Build history of the part. All positions in model axes, mm. Face numbers are marked on the shaded views. Give positions to 0.01 mm unless a question says otherwise; leave off trailing zeros. Write each loop counter-clockwise with the first axis right and the second up, starting at its lowest first coordinate (ties: lowest second). Pieces come first, ordered by that corner, then holes. Notation, with made-up numbers: M 9.25,58.25 L 28.25,58.25 A22 cw 28.25,64.25 Z; hole C 13.5,-10 d8. An arc over 180 degrees is marked long. One line per item, written item: value. Start each with the question number.
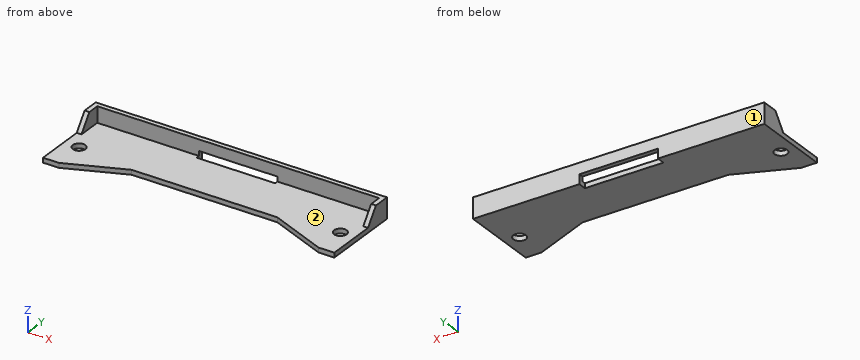
from build123d import *

# Parameters (mm, degrees)
SKETCH1_W           = 184
SKETCH1_H           = 50
SKETCH1_R           = 4
BOSS_EXTRUDE2_DEPTH = 3
SKETCH2_W           = 184
SKETCH2_H           = 3
BOSS_EXTRUDE3_DEPTH = 20
BOSS_EXTRUDE4_DEPTH = 3
BOSS_EXTRUDE5_DEPTH = 3
SKETCH5_W           = 49.622419658
SKETCH5_H           = 10.386730574
CUT_EXTRUDE3_DEPTH  = 6
SKETCH7_W           = 184
SKETCH7_H           = 10
CUT_EXTRUDE5_DEPTH  = 16
CUT_EXTRUDE7_DEPTH  = 16


with BuildPart() as part:
    # Sketch1 → Boss-Extrude2 (new body)
    with BuildSketch(Plane.XY):
        with Locations((92, 25)):
            Rectangle(SKETCH1_W, SKETCH1_H)
        with Locations((9.5, 20)):
            Circle(SKETCH1_R, mode=Mode.SUBTRACT)
        with Locations((174.5, 20)):
            Circle(SKETCH1_R, mode=Mode.SUBTRACT)
    extrude(amount=BOSS_EXTRUDE2_DEPTH)

    # Sketch2 → Boss-Extrude3 (add)
    with BuildSketch(Plane.XY.offset(3)):
        with Locations((92, 48.5)):
            Rectangle(SKETCH2_W, SKETCH2_H)
    extrude(amount=BOSS_EXTRUDE3_DEPTH)

    # Sketch3 → Boss-Extrude4 (add)
    with BuildSketch(Plane.ZY):
        Polygon((23, 47), (3, 47), (3, 32), align=None)
    extrude(amount=-BOSS_EXTRUDE4_DEPTH)

    # Sketch4 → Boss-Extrude5 (add)
    with BuildSketch(Plane(origin=(184, 0, 0), x_dir=(0, 0, -1), z_dir=(1, 0, 0))):
        Polygon((-23, 47), (-3, 32), (-3, 47), align=None)
    extrude(amount=-BOSS_EXTRUDE5_DEPTH)

    # Sketch5 → Cut-Extrude3 (cut)
    with BuildSketch(Plane(origin=(0, 0, 0), x_dir=(-1, 0, 0), z_dir=(0, 0, -1))):
        with Locations((-92, 50)):
            Rectangle(SKETCH5_W, SKETCH5_H)
    extrude(amount=-CUT_EXTRUDE3_DEPTH, mode=Mode.SUBTRACT)

    # Sketch7 → Cut-Extrude5 (cut)
    with BuildSketch(Plane(origin=(0, 50, 0), x_dir=(1, 0, 0), z_dir=(0, 1, 0))):
        with Locations((92, -18)):
            Rectangle(SKETCH7_W, SKETCH7_H)
    extrude(amount=-CUT_EXTRUDE5_DEPTH, mode=Mode.SUBTRACT)

    # Sketch8 → Cut-Extrude7 (cut)
    with BuildSketch(Plane.XY.offset(3)):
        Polygon((46, 15), (10, 0), (174, 0), (138, 15), align=None)
    extrude(amount=-CUT_EXTRUDE7_DEPTH, mode=Mode.SUBTRACT)


solid = part.part
1) Band-saw the part on D-D (y = 20). List the corners of the cut face in (x, z).
2) Band-saw the part on A-A (x = 77.5). List the corners of the cut face in (y, z), then the cut area to 3 significant figures.
3) Band-saw the part on B-B (y = 3). List the corners of the cut face in (x, z).
4) Band-saw the part on C-C (z = 8). List the corners of the cut face in (x, y), then the cut area to 4 significant figures.
5) Drop flat-ended pins along their axis: P1, Ø0.9, axis at x = 85.5, y = 48.5, coming from the -Z side; P2, Ø1.5, axis at x = 84, z = 1.5, coming from the +Y side; P3, Ø1.5, axis at x = 78.5, z = 1.5, coming from the -Y side; P4, Ø5, axis at x = 9.5, y = 20, coming from the +Z side. Give the stop position or say it passes through.
6) Mould opens along X. For the marked faces 1 and 2 say: released by +X, released by -X, zero draft, split by the parting line, or undercut.
7) Probe line 1 along Y through (x, z) = (174.5, 1.25); line 2 along X through (y, z) = (36, 4.25); line 3 along Z through (x, y) = (68, 28.5). List the from-to ranges inside material, lowest first. Write a range as from..to.
Model answer:
1. outline: M 0,0 L 5.5,0 L 5.5,3 L 0,3 Z; M 13.5,0 L 170.5,0 L 170.5,3 L 13.5,3 Z; M 178.5,0 L 184,0 L 184,3 L 178.5,3 Z
2. outline: M 15,0 L 44.81,0 L 44.81,3 L 15,3 Z; M 47,6 L 50,6 L 50,13 L 47,13 Z
2. area: 110 mm²
3. outline: M 0,0 L 17.2,0 L 17.2,3 L 0,3 Z; M 166.8,0 L 184,0 L 184,3 L 166.8,3 Z
4. outline: M 0,35.75 L 3,35.75 L 3,47 L 181,47 L 181,35.75 L 184,35.75 L 184,50 L 0,50 Z
4. area: 619.5 mm²
5. P1: stops at z = 6
5. P2: stops at y = 44.81
5. P3: stops at y = 15
5. P4: passes through
6. face 1: zero draft
6. face 2: undercut
7. line 1: y = 0..16, 24..50
7. line 2: x = 0..3, 181..184
7. line 3: z = 0..3
